The listing builds one solid part. Answer for the finished solid, in the listing's coordinates (mm). Face numbers are marked on the shaded views. A direction names the side the tool comes from. Give positions to 0.01 mm unless a question says otherwise; leave off trailing zeros. Order: outer loops, then holes, each group sorted by start corner. A loop starts at its lowest first (then second) coordinate and runs counter-clockwise, first axis right, second up. Notation, with made-up numbers: (24.25, -39.5) - (53.25, -39.5) arc R19 cw to (53.25, -17.5) - close; hole circle Ø5 at (-32.5, 62.25). An arc over 180 degrees is marked (long way). Use a Markdown table: item, result. Add a question column.
1) Flat-ended cylindrical pins translate along their axes: pin 1 (1.5 mm diameter, centred on y = -12, z = -2, fed in from -X); pin 2 (5.5 mm diameter, centred on x = 0, z = 0, fed in from -Y); pin 3 (1.2 mm diameter, centred on x = -3.5, y = -0.5, fed in from +Z); pin 4 (2.5 mm diameter, centred on x = -4.5, y = -1, fed in from -Z). Find the tip coordinate at first contact, or state that the pin passes through.
2) Find section B-B, the plane x = 1. Determine the outline of the cut face in (y, z), plus the area to 3 significant figures.
3) For the marked faces 4, 5, 6 and 7, determine the directions among +Z, -Z, +X, -X, +Y, -Y from which every point of the face is accessible in a straight line to the end or side of a thin tool.
4) The mould has two halves that part along Y. Classify the marked faces 1, 2 and 3: released by +Y, released by -Y, zero draft, split by the parting line, or undercut.
5) Straight lines are drawn through the part: line 1 (Y direction, x = -4.5, z = 1.5); line 2 (Y direction, x = 13, z = -1.75); line 3 (X direction, y = -6, z = 0). For each, find the intervals that lie inside material, in ascending order.
6) Find section A-A, the plane z = 0. State how many separate pieces and enclosed holes the cut face has, plus the area to 3 significant figures.
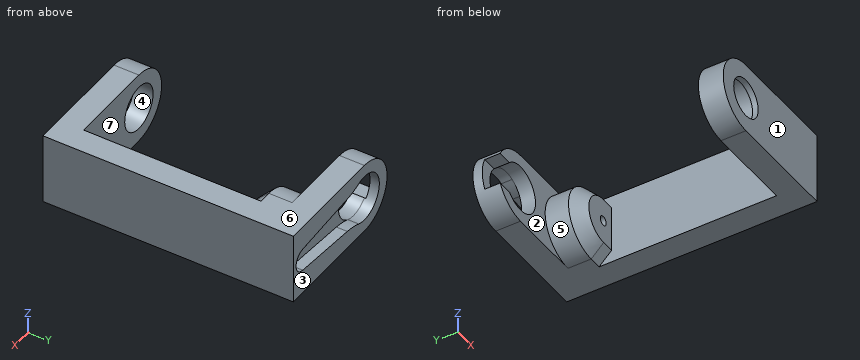
from build123d import *

# Parameters (mm, degrees)
SKETCH1_R                = 5.75
SKETCH1_R_2              = 3.8
BOSS_EXTRUDE1_DEPTH      = 2.25
BOSS_EXTRUDE2_DEPTH      = 2.25
SKETCH3_W                = 11.75
SKETCH3_H                = 11.5
BOSS_EXTRUDE3_DEPTH      = 5.75
BOSS_EXTRUDE4_START      = 1.75
BOSS_EXTRUDE4_DEPTH      = 1.75
FILLET3_R                = 10
SKETCH6_W                = 5.2
SKETCH6_H                = 2.5
CUT_EXTRUDE1_DEPTH       = 21.519807504
SKETCH7_R                = 0.75
CUT_EXTRUDE2_DEPTH       = 21.519807504
FILLET1_RADIUS           = 5.75
FILLET1_LENGTH           = 5.75
BOSS_EXTRUDE5_DEPTH      = 26.5
BOSS_EXTRUDE5_DEPTH_BACK = 4
SKETCH5_W                = 4
SKETCH5_H                = 11.5
CHAMFER1_SIZE            = 2
SKETCH8_R                = 3.6
BOSS_EXTRUDE6_DEPTH      = 4
BOSS_EXTRUDE7_START      = -0.9
SKETCH9_R                = 3.6
SKETCH9_R_2              = 3.1
BOSS_EXTRUDE7_DEPTH      = 0.9


with BuildPart() as part:
    # Sketch1 → Boss-Extrude1 (new body)
    with BuildSketch(Plane(origin=(0, 0, 0), x_dir=(1, 0, 0), z_dir=(0, 1, 0))):
        with Locations(Location((0, 0, 0), (0, 0, 270))):
            Circle(SKETCH1_R)
        with Locations(Location((0, 0, 0), (0, 0, 270))):
            Circle(SKETCH1_R_2, mode=Mode.SUBTRACT)
    extrude(amount=-BOSS_EXTRUDE1_DEPTH)

    # Sketch2 → Boss-Extrude2 (add)
    with BuildSketch(Plane(origin=(0, 0, 0), x_dir=(1, 0, 0), z_dir=(0, 1, 0))):
        with BuildLine():
            Line((0, 5.75), (18, 5.75))
            Line((18, 5.75), (18, -5.75))
            Line((18, -5.75), (0, -5.75))
            ThreePointArc((0, -5.75), (5.75, 0), (0, 5.75))
        make_face()
    extrude(amount=-BOSS_EXTRUDE2_DEPTH)

    # Sketch3 → Boss-Extrude3 (add)
    with BuildSketch(Plane.XZ.offset(2.25)):
        with Locations((12.125, 0)):
            Rectangle(SKETCH3_W, SKETCH3_H)
    extrude(amount=BOSS_EXTRUDE3_DEPTH)

    # Sketch4 → Boss-Extrude4 (add)
    with BuildSketch(Plane(origin=(0, 0, 0), x_dir=(1, 0, 0), z_dir=(0, 1, 0)).offset(BOSS_EXTRUDE4_START)):
        with BuildLine():
            Line((0, -5.75), (18, -5.75))
            Line((18, -5.75), (18, 5.75))
            Line((18, 5.75), (0, 5.75))
            ThreePointArc((0, 5.75), (-5.75, 0), (0, -5.75))
        make_face()
        with BuildLine():
            Line((2.336179457, -2.9970428), (15.610227504, -1.84304833))
            ThreePointArc((15.610227504, -1.84304833), (17.3, 0), (15.610227504, 1.84304833))
            Line((15.610227504, 1.84304833), (2.336179457, 2.9970428))
            ThreePointArc((2.336179457, 2.9970428), (-3.8, 0), (2.336179457, -2.9970428))
        make_face(mode=Mode.SUBTRACT)
    extrude(amount=-BOSS_EXTRUDE4_DEPTH)

    # Fillet3
    # the kernel refuses this fillet: 10 mm, written as the material it takes off along each edge
    with BuildSketch(Plane(origin=(2.336179457, 6.739658122, 2.9970428), x_dir=(-0.8658918638658896, 0, 0.5002312266251037), z_dir=(0, -1, 0))) as fillet3_piece_1:
        with BuildLine():
            CenterArc((2.425392956, -9.90459182), FILLET3_R, 97.920932923, 17.12578451)
            Line((-1.808178045, -0.844962877), (0, 0))
            ThreePointArc((0, 0), (0.523664388, -0.036255108), (1.047328776, 0))
        make_face()
    extrude(amount=6.739658122, mode=Mode.SUBTRACT)
    with BuildSketch(Plane(origin=(2.336179457, 6.739658122, -2.9970428), x_dir=(-0.8658918638659203, 0, -0.5002312266250502), z_dir=(0, -1, 0))) as fillet3_piece_2:
        with BuildLine():
            CenterArc((2.425392956, 9.90459182), FILLET3_R, 244.953282566, 17.12578451)
            Line((-1.808178045, 0.844962877), (0, 0))
            ThreePointArc((0, 0), (0.523664388, 0.036255108), (1.047328776, 0))
        make_face()
    extrude(amount=6.739658122, mode=Mode.SUBTRACT)

    # Sketch6 → Cut-Extrude1 (cut, through all)
    with BuildSketch(Plane(origin=(0, 0, 0), x_dir=(0, 0, -1), z_dir=(1, 0, 0))):
        with Locations((0, -1)):
            Rectangle(SKETCH6_W, SKETCH6_H)
    extrude(amount=-CUT_EXTRUDE1_DEPTH, mode=Mode.SUBTRACT)

    # Sketch7 → Cut-Extrude2 (cut, through all)
    with BuildSketch(Plane(origin=(0, 0, 0), x_dir=(1, 0, 0), z_dir=(0, 1, 0))):
        with Locations(Location((11.91, 0, 0), (0, 0, 270))):
            Circle(SKETCH7_R)
    extrude(amount=-CUT_EXTRUDE2_DEPTH, mode=Mode.SUBTRACT)

    # Fillet1: full round fillet: the end face becomes a half cylinder, R = half its width
    fillet1_face = Plane((6.25, -5.125, 0), x_dir=(0, -1, 0), z_dir=(-1, 0, 0))  # on the end face: x along it, z out of the body
    fillet1_slab = fillet1_face.offset(-FILLET1_RADIUS / 2) * Box(FILLET1_LENGTH, 2 * FILLET1_RADIUS, FILLET1_RADIUS, mode=Mode.PRIVATE)  # the body's end, R deep
    fillet1_round = Plane((12, -5.125, 0), x_dir=(-1, 0, 0), z_dir=(0, -1, 0)) * Cylinder(FILLET1_RADIUS, FILLET1_LENGTH, mode=Mode.PRIVATE)  # its axis R under the face
    add(fillet1_slab - fillet1_round, mode=Mode.SUBTRACT)

    # Sketch5 → Boss-Extrude5 (add, two sides: drawn at the far end of the back side and taken through both)
    with BuildSketch(Plane.XZ.offset(8).offset(-BOSS_EXTRUDE5_DEPTH_BACK)):
        with Locations((16, 0)):
            Rectangle(SKETCH5_W, SKETCH5_H)
    extrude(amount=BOSS_EXTRUDE5_DEPTH + BOSS_EXTRUDE5_DEPTH_BACK)

    # Chamfer1
    chamfer1_edges = [part.edges().sort_by_distance(p)[0] for p in [
        (6.25, -8, 0),
        (13, -8, 5.75),
        (13, -8, -5.75),
    ]]
    chamfer(chamfer1_edges, length=CHAMFER1_SIZE)

    # Sketch8 → Boss-Extrude6 (add)
    with BuildSketch(Plane.XZ.offset(34.5)):
        with BuildLine():
            Line((18, 5.75), (0, 5.75))
            ThreePointArc((0, 5.75), (-5.75, 0), (0, -5.75))
            Line((0, -5.75), (18, -5.75))
            Line((18, -5.75), (18, 5.75))
        make_face()
        with Locations(Location((0, 0, 0), (0, 0, 270))):
            Circle(SKETCH8_R, mode=Mode.SUBTRACT)
    extrude(amount=BOSS_EXTRUDE6_DEPTH)

    # Sketch9 → Boss-Extrude7 (add)
    with BuildSketch(Plane.XZ.offset(38.5).offset(BOSS_EXTRUDE7_START)):
        with Locations(Location((0, 0, 0), (0, 0, 270))):
            Circle(SKETCH9_R)
        with Locations(Location((0, 0, 0), (0, 0, 270))):
            Circle(SKETCH9_R_2, mode=Mode.SUBTRACT)
    extrude(amount=BOSS_EXTRUDE7_DEPTH)


solid = part.part
The answers:
| question | item | result |
|---|---|---|
| 1 | pin 1 | x = 14 |
| 1 | pin 2 | through |
| 1 | pin 3 | z = 4.97 |
| 1 | pin 4 | z = -4.74 |
| 2 | outline | (-38.5, -5.75) - (-34.5, -5.75) - (-34.5, -3.46) - (-37.6, -3.46) - (-37.6, -2.93) - (-38.5, -2.93) - close; (-38.5, 2.93) - (-37.6, 2.93) - (-37.6, 3.46) - (-34.5, 3.46) - (-34.5, 5.75) - (-38.5, 5.75) - close; (-2.25, -5.75) - (1.75, -5.75) - (1.75, -3.67) - (-2.25, -3.67) - close; (-2.25, 3.67) - (1.75, 3.67) - (1.75, 5.75) - (-2.25, 5.75) - close |
| 2 | area | 35.9 mm2 |
| 3 | face 4 | +Y |
| 3 | face 5 | -X |
| 3 | face 6 | +Z, +X, -X, +Y, -Y |
| 3 | face 7 | +Z, -Z, -X |
| 4 | face 1 | released by -Y |
| 4 | face 2 | undercut |
| 4 | face 3 | released by +Y |
| 5 | line 1 | -38.5 to -34.5, 0.25 to 1.75 |
| 5 | line 2 | -38.5 to -34.5, -8 to 0 |
| 5 | line 3 | 6.25 to 11.16, 12.66 to 18 |
| 6 | separate pieces | 4 |
| 6 | enclosed holes | 0 |
| 6 | area | 263 mm2 |
